Geometry check sheet. Reference: drawing and pictorial views, mm from the part's lowest x, y, z. Round coordinates to 2 decimals unless told otherwise and drop trailing zeros. Order: outer loops, then holes, each group sorted by start corner. A loop starts at its lowest first (then second) coordinate and runs counter-clockwise, first axis right, second up.
(1) Sectioned sample at C-C, the plane y = 95. Enter the section's corners in (x, z).
(2) Sectioned sample at A-A, the plane y = 45. Enter the section's corners in (x, z).
(3) Depth check by flat-ended pin: pin 1 (4.5 mm diameter, centred on x = 160, y = 20, fed in from -Z); pin 2 (1.5 mm diameter, centred on x = 144.5, z = 2, fed in from +Y); pin 3 (1 mm diameter, centred on x = 145, z = 0.5, fed in from +Y); pin 4 (3 mm diameter, centred on x = 51.5, z = 2, fed in from +Y) (1 decimal). Enter the tip coordinate at first touch or a pass-through.
(4) Thickness scan on probe 1 along Y at (x, z) = (85, 1.95); probe 2 along Y at (x, z) = (160, 3.2); probe 3 along Y at (x, z) = (76.5, 4.3) (1 decimal). Record the ranges inside material, lowest first.
(5) Sectioned sample at B-B, the plane x = 10. Enter the section's corners in (y, z).
(6) Sectioned sample at D-D, the plane z = 1.4. Enter the section's corners in (x, y).
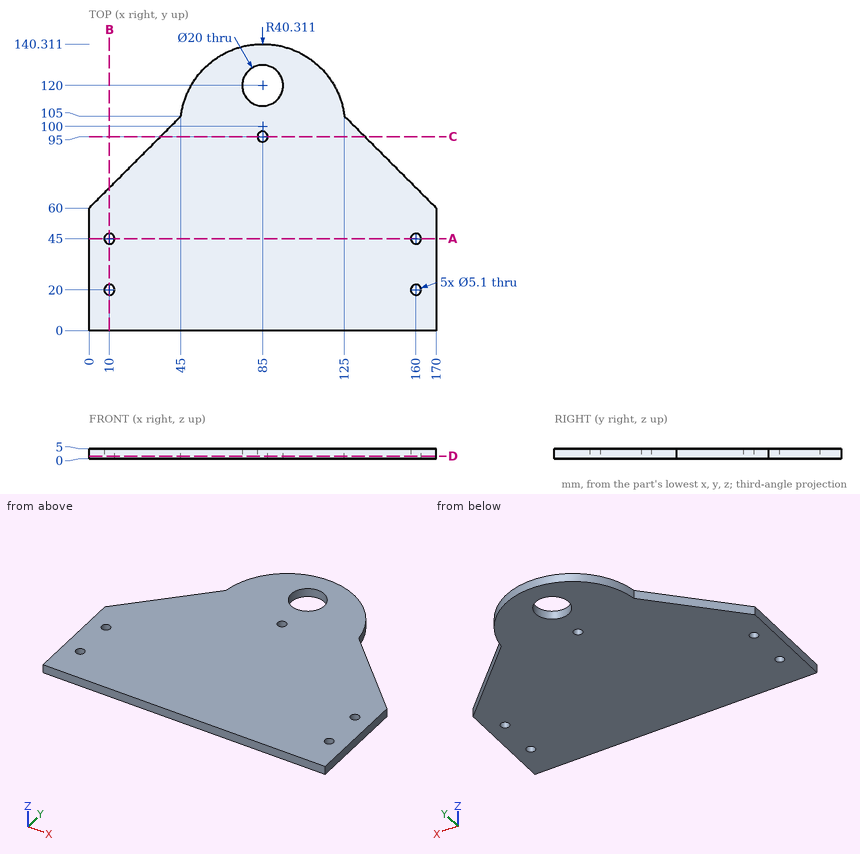
Derived:
1. outline: (35, 0) - (82.45, 0) - (82.45, 5) - (35, 5) - close; (87.55, 0) - (135, 0) - (135, 5) - (87.55, 5) - close
2. outline: (0, 0) - (7.45, 0) - (7.45, 5) - (0, 5) - close; (12.55, 0) - (157.45, 0) - (157.45, 5) - (12.55, 5) - close; (162.55, 0) - (170, 0) - (170, 5) - (162.55, 5) - close
3. pin 1: passes through
3. pin 2: stops at y = 86.25
3. pin 3: stops at y = 85.5
3. pin 4: stops at y = 124.5
4. probe 1: y = 0 to 92.45, 97.55 to 110, 130 to 140.31
4. probe 2: y = 0 to 17.45, 22.55 to 42.45, 47.55 to 70
4. probe 3: y = 0 to 114.7, 125.3 to 139.4
5. outline: (0, 0) - (17.45, 0) - (17.45, 5) - (0, 5) - close; (22.55, 0) - (42.45, 0) - (42.45, 5) - (22.55, 5) - close; (47.55, 0) - (70, 0) - (70, 5) - (47.55, 5) - close
6. outline: (0, 0) - (170, 0) - (170, 60) - (125, 105) arc R40.31 ccw to (45, 105) - (0, 60) - close; hole circle Ø5.1 at (10, 20); hole circle Ø5.1 at (10, 45); hole circle Ø20 at (85, 120); hole circle Ø5.1 at (85, 95); hole circle Ø5.1 at (160, 20); hole circle Ø5.1 at (160, 45)
